Could you check a few things on this model? Use its own coordinates, in mm. Face numbers are marked on the shaded views. Give positions to 0.01 mm unless a question says otherwise; leave off trailing zeros. Write each loop counter-clockwise with the first axis right and the second up, starting at its lowest first coordinate (ties: lowest second). Pieces come first, ordered by that corner, then holes. Notation, with made-up numbers: M 37,63 L 70,63 A31 ccw 70,97 Z; hole C 64,85.25 d9. An arc over 180 degrees is marked long. Write each question's results on one line, items separated by ' | '. Start each with the question number.
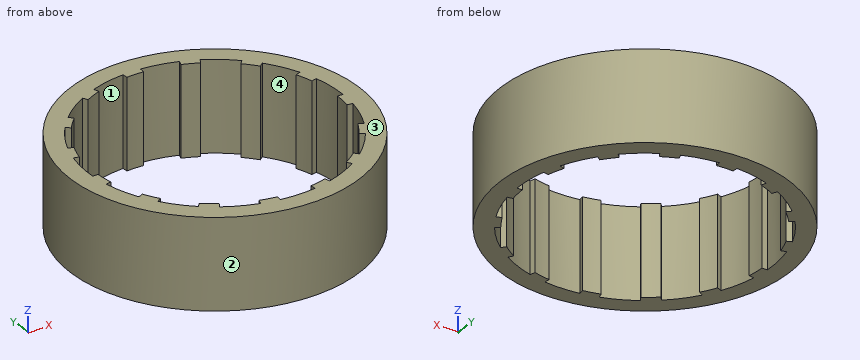
Autodesk Inventor part; units mm, degrees
ref_plane "YZ Plane" through (0, 0, 0) normal (1, 0, 0) x (0, 1, 0)
ref_plane "XZ Plane" through (0, 0, 0) normal (0, 1, 0) x (-1, 0, 0)
ref_plane "XY Plane" through (0, 0, 0) normal (0, 0, 1) x (1, 0, 0)
sketch "Sketch1" plane through (0, 0, 0) normal (0, 0, 1) x (1, 0, 0)
  circle A0 centre (0, 0) radius 20.32
  circle A1 centre (0, 0) radius 17.78
  arc A2 (1.1871, 16.9765) -> (-1.1871, 16.9765) centre (0, 0) ccw
  line L0 (0, 17.018) -> (0, 20.32)
  line L1 (1.1871, 16.9765) -> (1.2403, 17.7367)
  line L2 (-1.1871, 16.9765) -> (-1.2403, 17.7367)
  dimension "d0" = 40.64
  dimension "d1" = 2.54
  dimension "d2" = 0.762
  dimension "d3" = 4
  dimension "d4" = 4
extrude "Extrusion1" add sketch "Sketch1" along normal blind 12.7 contours A1 L1 A2 L0 | L0 A2 L2 A1 | A0
pattern_circular "Circular Pattern1" count 15 over 360 about axis through (0, 0, 0) along (0, 0, 1) of "Extrusion1"
properties part number "RubberWheelNT"
Q1. If we section it at B-B (y = 0): Please give me the cut outline in (x, z).
Q2. If we mould it in two halves opening along X, with no side actions, what happens to the marked faces 1, 2, 3 and 4? For each: pulls with the +X half, pulls with the -X half, needs draft (parallel to the pull), parting line crosses it, or undercut.
Q3. I'm going to push flat-ended pins straight in: P1, Ø2, axis at x = 14, y = -13.5, coming from the -Z side; P2, Ø4, axis at x = 6, y = 12.5, coming from the +Z side; P3, Ø4, axis at y = -13.5, z = 5.5, coming from the +X side; P4, Ø1, axis at y = 3, z = 11, coming from the +X side. Where does each tip first touch, or does it pass through?
Q4. If we section it at A-A (x = 0): Please give me the cut outline in (y, z).
Q5. Please list where these lines run through material, in increasing order: line 1 (X direction, y = 15.5, z = 8.75); line 2 (X direction, y = 3.5, z = 2); line 3 (Y direction, x = -1, z = 4). Write a range as [from, to].
Determined:
1) outline: M -20.32,0 L -17.78,0 L -17.78,12.7 L -20.32,12.7 Z; M 17.78,0 L 20.32,0 L 20.32,12.7 L 17.78,12.7 Z
2) face 1: undercut | face 2: parting line crosses it | face 3: needs draft | face 4: undercut
3) P1: stops at z = 0 | P2: passes through | P3: stops at x = 16.75 | P4: stops at x = 20.17
4) outline: M -20.32,0 L -17.78,0 L -17.78,12.7 L -20.32,12.7 Z; M 17.02,0 L 20.32,0 L 20.32,12.7 L 17.02,12.7 Z
5) line 1: x = [-13.14, -8.71], [-8.24, -7.03], [7.03, 8.24], [8.71, 13.14] | line 2: x = [-20.02, -17.43], [17.43, 20.02] | line 3: y = [-20.3, -17.75], [16.99, 20.3]
